Geometry: final body of the model. Coordinates: model frame, mm. Coordinates: 2 decimals unless noted, no trailing zeros. Write each loop counter-clockwise with the first axis right and the second up, starting at its lowest first coordinate (ties: lowest second). Pieces come first, ordered by that corner, then holes. Notation, with made-up numbers: M 79,13 L 104,13 A21 cw 104,48 Z; hole C 12,-30.5 d11. An arc over 180 degrees is marked long. Write item = value, one per line. Start each with the question number.
Item 1: Section A-A on x = 0. Output: boundary loops of the cut face in (y, z), plus the area to 3 significant figures.
Item 2: Section C-C on z = 4. Output: boundary loops of the cut face in (x, y).
Item 3: Ray query, L1, parallel to Y at x = 0, z = -9.65; L2, parallel to Z at x = 3.75, y = 117. Return the intervals inside material, ascending. Write a range as [from, to].
Item 4: Section B-B on y = 26.5. Output: boundary loops of the cut face in (x, z).
from build123d import *

# Parameters (mm, degrees)
F0_W     = 20
F0_H     = 20
F0_W_2   = 18.2
F0_H_2   = 18.2
F1_DEPTH = 175
F2_R     = 1
F4_D     = 8.5


with BuildPart() as f1:
    # F0 (on Front) → F1 (new body, symmetric)
    with BuildSketch(Plane.XZ):
        Rectangle(F0_W, F0_H)
        Rectangle(F0_W_2, F0_H_2, mode=Mode.SUBTRACT)
    extrude(amount=F1_DEPTH, both=True)

    # F2
    f2_edges = [f1.edges().sort_by_distance(p)[0] for p in [
        (10, 0, 10),
        (-10, 0, 10),
        (10, 0, -10),
        (-10, 0, -10),
    ]]
    fillet(f2_edges, radius=F2_R)

    # F4 (through all)
    with Locations(Plane.XY.offset(10)):
        with Locations((0, -13.331), (0, -106.669)):
            Hole(F4_D / 2)


solid = f1.part
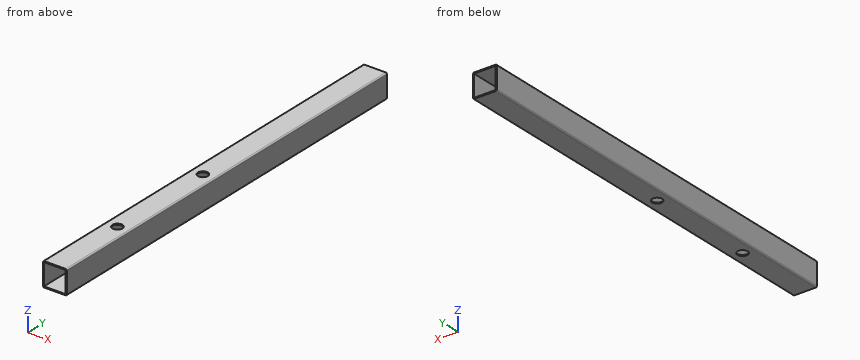
Responses:
q1.outline = M -175,-10 L -110.92,-10 L -110.92,-9.1 L -175,-9.1 Z; M -175,9.1 L -110.92,9.1 L -110.92,10 L -175,10 Z; M -102.42,-10 L -17.58,-10 L -17.58,-9.1 L -102.42,-9.1 Z; M -102.42,9.1 L -17.58,9.1 L -17.58,10 L -102.42,10 Z; M -9.08,-10 L 175,-10 L 175,-9.1 L -9.08,-9.1 Z; M -9.08,9.1 L 175,9.1 L 175,10 L -9.08,10 Z
q1.area = 599 mm²
q2.outline = M -10,-175 L -9.1,-175 L -9.1,175 L -10,175 Z; M 9.1,-175 L 10,-175 L 10,175 L 9.1,175 Z
q3.L1 = [-175, -110.92], [-102.42, -17.58], [-9.08, 175]
q3.L2 = [-10, -9.1], [9.1, 10]
q4.outline = M -10,-9 A1 ccw -9,-10 L 9,-10 A1 ccw 10,-9 L 10,9 A1 ccw 9,10 L -9,10 A1 ccw -10,9 Z; hole M -9.1,-9.1 L 9.1,-9.1 L 9.1,9.1 L -9.1,9.1 Z
